```python
from build123d import *

# Parameters (mm, degrees)
SKETCH1_W           = 160
SKETCH1_H           = 50
BOSS_EXTRUDE1_DEPTH = 2.5
SKETCH2_R           = 3.75
CUT_EXTRUDE1_DEPTH  = 168.649187293
SKETCH3_W           = 160
SKETCH3_H           = 50
SKETCH3_W_2         = 156
SKETCH3_H_2         = 46
BOSS_EXTRUDE2_DEPTH = 30
SKETCH5_W           = 160
SKETCH5_H           = 2.049984413
BOSS_EXTRUDE4_DEPTH = 15
BOSS_EXTRUDE5_DEPTH = 2
BOSS_EXTRUDE7_DEPTH = 2
SKETCH9_R           = 5
CUT_EXTRUDE2_DEPTH  = 3


with BuildPart() as part:
    # Sketch1 → Boss-Extrude1 (new body)
    with BuildSketch(Plane(origin=(0, 0, 0), x_dir=(1, 0, 0), z_dir=(0, 1, 0))):
        with Locations((80, -25)):
            Rectangle(SKETCH1_W, SKETCH1_H)
    extrude(amount=BOSS_EXTRUDE1_DEPTH)

    # Sketch2 → Cut-Extrude1 (cut, through all)
    with BuildSketch(Plane(origin=(0, 2.5, 0), x_dir=(1, 0, 0), z_dir=(0, 1, 0))):
        with Locations(Location((15, -25, 0), (0, 0, 270))):
            Circle(SKETCH2_R)
        with Locations(Location((36, -25, 0), (0, 0, 270))):
            Circle(SKETCH2_R)
        with Locations(Location((57, -25, 0), (0, 0, 270))):
            Circle(SKETCH2_R)
        with Locations(Location((78, -25, 0), (0, 0, 270))):
            Circle(SKETCH2_R)
        with Locations(Location((99, -25, 0), (0, 0, 270))):
            Circle(SKETCH2_R)
        with Locations(Location((120, -25, 0), (0, 0, 270))):
            Circle(SKETCH2_R)
        with Locations(Location((141, -25, 0), (0, 0, 270))):
            Circle(SKETCH2_R)
    extrude(amount=-CUT_EXTRUDE1_DEPTH, mode=Mode.SUBTRACT)

    # Sketch3 → Boss-Extrude2 (add)
    with BuildSketch(Plane(origin=(0, 2.5, 0), x_dir=(1, 0, 0), z_dir=(0, 1, 0))):
        with Locations((80, -25)):
            Rectangle(SKETCH3_W, SKETCH3_H)
        with Locations((80, -25)):
            Rectangle(SKETCH3_W_2, SKETCH3_H_2, mode=Mode.SUBTRACT)
    extrude(amount=BOSS_EXTRUDE2_DEPTH)

    # Sketch5 → Boss-Extrude4 (add)
    with BuildSketch(Plane(origin=(0, 32.5, 0), x_dir=(1, 0, 0), z_dir=(0, 1, 0))):
        with Locations((80, -1.024992207)):
            Rectangle(SKETCH5_W, SKETCH5_H)
    extrude(amount=BOSS_EXTRUDE4_DEPTH)

    # Sketch6 → Boss-Extrude5 (add)
    with BuildSketch(Plane(origin=(160, 0, 0), x_dir=(0, 0, -1), z_dir=(1, 0, 0))):
        Polygon((-2.049984413, 32.5), (-50, 32.5), (-2.049984413, 47.5), align=None)
    extrude(amount=-BOSS_EXTRUDE5_DEPTH)

    # Sketch8 → Boss-Extrude7 (add)
    with BuildSketch(Plane.ZY):
        Polygon((2.049984413, 47.5), (2.049984413, 32.5), (50, 32.5), align=None)
    extrude(amount=-BOSS_EXTRUDE7_DEPTH)

    # Sketch9 → Cut-Extrude2 (cut)
    with BuildSketch(Plane(origin=(0, 0, 0), x_dir=(-1, 0, 0), z_dir=(0, 0, -1))):
        with Locations((-80, 31.153444526)):
            Circle(SKETCH9_R)
    extrude(amount=-CUT_EXTRUDE2_DEPTH, mode=Mode.SUBTRACT)


solid = part.part
```
Input: part model. Units: mm. Frame: model coordinates. A direction names the side the tool comes from. Round coordinates to 2 decimals unless told otherwise and drop trailing zeros. Loops run counter-clockwise (first coordinate to the right, second up) from the corner with the lowest first, then second, coordinate; pieces in that order, holes last. Notation, with made-up numbers: (-28.5, -8) - (-2.5, -8) arc R33 cw to (-2.5, 25) - close; hole circle Ø6 at (42, 81.25). An arc over 180 degrees is marked (long way). One line per item, written item: value. Start each with the question number.
(1) Draft query along X for faces 4 (the flat face through (160, 19, 25)), 5 (the flat face through (79, 23, 0)), 6 (the cylindrical face through (102.718, 1.268, 24.512)). Return one class per face: +X half, -X half, draft (parallel to the pull), parting line (faces both ways), or undercut.
(2) Ray query, line 1 (Z direction, x = 54, y = 17.5); line 2 (X direction, y = 40, z = 15); line 3 (Y direction, x = 80, z = 1). Return the intervals inside material, ascending. Write a range as [from, to].
(3) Contact query for flat-ended pins moving along their axis: P1, Ø8.5, axis at x = 36, z = 25, coming from the +Y side; P2, Ø7, axis at x = 141, z = 25, coming from the -Y side; P3, Ø2, axis at x = 45, y = 35.5, coming from the +Z side; P4, Ø9, axis at x = 80, y = 31.15, coming from the -Z side. Output: stop coordinate, or through.
(4) Section C-C, the plane y = 34. Return loops of the section in (x, z) (3 decimals).
(5) Section A-A, the plane y = 15.5. Return loops of the section in (x, z).
(6) Section B-B, the plane x = 36. Return loops of the section in (y, z).
(7) Access query for faces 1 (the cylindrical face through (53.673, 1.268, 26.73)), 2 (the flat face through (79, 40, 2.05)), 3 (the flat face through (79, 17, 48)). Directions: +Z, -Z, +X, -X, +Y, -Y. A direction counts if a zero-diameter tool reaches every point of the face in a straight line with its end or side. Return the directions, or none.
(8) Section D-D, the plane z = 15.5. Return loops of the section in (x, y), plus the area to 3 significant figures.
Results below:
1. face 4: +X half
1. face 5: draft
1. face 6: undercut
2. line 1: [0, 2], [48, 50]
2. line 2: [0, 2], [158, 160]
2. line 3: [0, 26.15], [36.15, 47.5]
3. P1: y = 2.5
3. P2: through
3. P3: z = 2.05
3. P4: z = 48
4. outline: (0, 0) - (75.889, 0) - (75.889, 2.05) - (2, 2.05) - (2, 45.205) - (0, 45.205) - close; (84.111, 0) - (160, 0) - (160, 45.205) - (158, 45.205) - (158, 2.05) - (84.111, 2.05) - close
5. outline: (0, 0) - (160, 0) - (160, 50) - (0, 50) - close; hole (2, 2) - (158, 2) - (158, 48) - (2, 48) - close
6. outline: (0, 0) - (47.5, 0) - (47.5, 2.05) - (32.5, 2.05) - (32.5, 2) - (2.5, 2) - (2.5, 21.25) - (0, 21.25) - close; (0, 28.75) - (2.5, 28.75) - (2.5, 48) - (32.5, 48) - (32.5, 50) - (0, 50) - close
7. face 1: +Y, -Y
7. face 2: +Z, +Y
7. face 3: +Y
8. outline: (0, 0) - (160, 0) - (160, 43.29) - (158, 43.29) - (158, 2.5) - (2, 2.5) - (2, 43.29) - (0, 43.29) - close
8. area: 563 mm^2
